from build123d import *

# Parameters (mm, degrees)
SKETCH_W             = 133
SKETCH_H             = 90
PAD_DEPTH            = 10
PAD001_DEPTH         = 24
PAD002_DEPTH         = 133
SKETCH003_W          = 101
SKETCH003_H          = 2
PAD003_DEPTH         = 36
SKETCH004_W          = 2
SKETCH004_H          = 3
PAD004_DEPTH         = 30
LINEARPATTERN_COUNT  = 6
LINEARPATTERN_PITCH  = 16.6
SKETCH005_W          = 100
SKETCH005_H          = 55
POCKET_DEPTH         = 6
SKETCH006_W          = 94
SKETCH006_H          = 49
POCKET001_DEPTH      = 36.001
SKETCH007_W          = 6
SKETCH007_H          = 6
POCKET002_DEPTH      = 57
POCKET002_DEPTH_BACK = -57
FILLET_R             = 3
FILLET001_R          = 3
CHAMFER_SIZE         = 1
SKETCH008_W          = 3
SKETCH008_H          = 55
PAD005_DEPTH         = 3
FILLET002_R          = 2
FILLET003_R          = 2


with BuildPart() as part:
    # Sketch → Pad (new body)
    with BuildSketch(Plane.XY):
        with Locations((0, 5)):
            Rectangle(SKETCH_W, SKETCH_H)
    extrude(amount=PAD_DEPTH)

    # Sketch001 → Pad001 (join)
    with BuildSketch(Plane.XY):
        with BuildLine():
            Line((-66.5, -40), (-66.5, 50))
            Line((-66.5, 50), (-54, 50))
            Line((-54, 50), (-54, 48))
            Line((-54, 48), (-57, 48))
            Line((-57, 48), (-57, 42))
            Line((-57, 42), (-54, 42))
            Line((-54, 42), (-54, 40))
            Line((-54, 40), (-57, 40))
            Line((-57, 40), (-57, -32))
            Line((-57, -32), (-55.06066, -33.93934))
            ThreePointArc((-55.06066, -36.06066), (-54.62132, -35), (-55.06066, -33.93934))
            Line((-55.06066, -36.06066), (-57, -38))
            Line((-57, -38), (-57, -40))
            Line((-57, -40), (-66.5, -40))
        make_face()
    pad001 = extrude(amount=PAD001_DEPTH)

    # Mirrored: Pad001 across Sketch001 V_Axis
    add(pad001.mirror(Plane(origin=(0, 0, 0), x_dir=(0, 0, 1), z_dir=(1, 0, 0))))

    # Sketch002 (on Face10 of Mirrored) → Pad002 (join)
    with BuildSketch(Plane(origin=(-66.5, 0, 0), x_dir=(0, -1, 0), z_dir=(-1, 0, 0))):
        with BuildLine():
            Line((32, 10), (33.93934, 11.93934))
            ThreePointArc((36.06066, 11.93934), (35, 12.37868), (33.93934, 11.93934))
            Line((36.06066, 11.93934), (38, 10))
            Line((38, 10), (32, 10))
        make_face()
    extrude(amount=-PAD002_DEPTH)

    # Sketch003 → Pad003 (join)
    with BuildSketch(Plane.XY):
        with Locations((0, -26.5)):
            Rectangle(SKETCH003_W, SKETCH003_H)
    extrude(amount=PAD003_DEPTH)

    # Sketch004 → Pad004 (join)
    with BuildSketch(Plane.XY):
        with Locations((41.6, -24.5)):
            Rectangle(SKETCH004_W, SKETCH004_H)
    pad004 = extrude(amount=PAD004_DEPTH)

    # LinearPattern: Pad004 ×6
    with Locations(*[(-i * LINEARPATTERN_PITCH, 0, 0) for i in range(1, LINEARPATTERN_COUNT)]):
        add(pad004)

    # Sketch005 (on Face38 of LinearPattern) → Pocket (cut)
    with BuildSketch(Plane.XY.offset(10)):
        with Locations((0, 7.5)):
            Rectangle(SKETCH005_W, SKETCH005_H)
    extrude(amount=-POCKET_DEPTH, mode=Mode.SUBTRACT)

    # Sketch006 → Pocket001 (cut, through all)
    with BuildSketch(Plane.XY):
        with Locations((0, 7.5)):
            Rectangle(SKETCH006_W, SKETCH006_H)
    extrude(amount=POCKET001_DEPTH, mode=Mode.SUBTRACT)

    # Sketch007 → Pocket002 (cut, two sides)
    with BuildSketch(Plane.YZ) as pocket002_sk:
        with Locations((45, 8)):
            Rectangle(SKETCH007_W, SKETCH007_H)
    extrude(amount=-POCKET002_DEPTH, mode=Mode.SUBTRACT)
    extrude(pocket002_sk.sketch, amount=-POCKET002_DEPTH_BACK, mode=Mode.SUBTRACT)

    # Fillet
    fillet_edges = [part.edges().sort_by_distance(p)[0] for p in [
        (-66.5, -40, 17),
        (-66.5, -40, 5),
        (-66.5, 50, 17),
        (-66.5, 50, 5),
    ]]
    fillet(fillet_edges, radius=FILLET_R)

    # Fillet001
    fillet001_edges = [part.edges().sort_by_distance(p)[0] for p in [
        (66.5, 50, 17),
        (66.5, 50, 5),
        (66.5, -40, 17),
        (66.5, -40, 5),
    ]]
    fillet(fillet001_edges, radius=FILLET001_R)

    # Chamfer
    chamfer_edges = [part.edges().sort_by_distance(p)[0] for p in [
        (66.5, 5, 0),
        (65.62132, 49.12132, 0),
        (58.75, 50, 0),
        (0, 50, 0),
        (-58.75, 50, 0),
        (-65.62132, 49.12132, 0),
        (-66.5, 5, 0),
        (-65.62132, -39.12132, 0),
        (-60.25, -40, 0),
        (0, -40, 0),
        (60.25, -40, 0),
        (65.62132, -39.12132, 0),
    ]]
    chamfer(chamfer_edges, length=CHAMFER_SIZE)

    # Sketch008 (on Face13 of Chamfer) → Pad005 (join)
    with BuildSketch(Plane.XY.offset(24)):
        with Locations((58.5, 7.5)):
            Rectangle(SKETCH008_W, SKETCH008_H)
        with Locations((-58.5, 7.5)):
            Rectangle(SKETCH008_W, SKETCH008_H)
    extrude(amount=PAD005_DEPTH)

    # Fillet002
    fillet002_edges = [part.edges().sort_by_distance(p)[0] for p in [
        (60, -20, 25.5),
        (60, 35, 25.5),
    ]]
    fillet(fillet002_edges, radius=FILLET002_R)

    # Fillet003
    fillet003_edges = [part.edges().sort_by_distance(p)[0] for p in [
        (-60, -20, 25.5),
        (-60, 35, 25.5),
    ]]
    fillet(fillet003_edges, radius=FILLET003_R)


solid = part.part
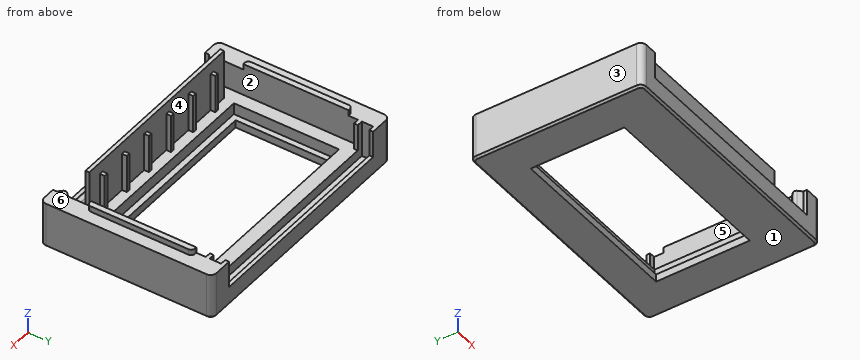
Could you check a few things on this model? Use its own coordinates, in mm. Face numbers are marked on the shaded views. A direction names the side the tool comes from. Coordinates: 2 decimals unless noted, no trailing zeros. Order: outer loops, then holes, each group sorted by start corner. A loop starts at its lowest first (then second) coordinate and runs counter-clockwise, first axis right, second up. Notation, with made-up numbers: (86.25, -22.5) -> (103.25, -22.5) arc R23 cw to (103.25, -14.5) -> close; hole circle Ø3 at (13, 8.25). An arc over 180 degrees is marked (long way). One line per item, written item: value. Start each with the question number.
1) Imagine slicing it at B-B on y = 19. List the corners of the cut face in (x, z) for me.
2) Which directions (+Z, -Z, +X, -X, +Y, -Y) give clear straight access to the entire face, cutting with the end or side of a thin tool? Please do the marked faces 1 and 2.
3) We'd pull the mould along X, two halves only. Please class the marked faces 3, 4, 5 and 6: +X half, -X half, draft (parallel to the pull), parting line (faces both ways), or undercut.
4) I'm going to push flat-ended pins straight in: pin 1 (0.8 mm diameter, centred on x = 57.5, z = 26, fed in from +Y); pin 2 (0.9 mm diameter, centred on x = -58.5, y = 8.5, fed in from +Z); pin 3 (1 mm diameter, centred on x = -41, z = 18.5, fed in from +Y). Where does each tip first touch, or does it pass through?
5) Imagine slicing it at D-D on y = -21.5. List the corners of the cut face in (x, z) for me.
6) Imagine slicing it at C-C on z = 8.5. List the corners of the cut face in (x, y) for me.
7) If I drill on L1, parallel to X at y = -27, z = 22; L2, parallel to X at y = 38.5, z = 22; L3, parallel to X at y = -25, z = 26.5, over which ranges is the centre line in solid material (lowest first)? Write a range as [from, to].
8) Imagine slicing it at A-A on x = 34. List the corners of the cut face in (y, z) for me, plus the area to 3 significant figures.
Answer list:
1. outline: (-66.5, 1) -> (-65.5, 0) -> (-47, 0) -> (-47, 4) -> (-50, 4) -> (-50, 10) -> (-57, 10) -> (-57, 27) -> (-60, 27) -> (-60, 24) -> (-66.5, 24) -> close; (47, 0) -> (65.5, 0) -> (66.5, 1) -> (66.5, 24) -> (60, 24) -> (60, 27) -> (57, 27) -> (57, 10) -> (50, 10) -> (50, 4) -> (47, 4) -> close
2. face 1: -Z, +X, -X, +Y, -Y
2. face 2: +Z
3. face 3: -X half
3. face 4: undercut
3. face 5: undercut
3. face 6: draft
4. pin 1: stops at y = 35
4. pin 2: stops at z = 27
4. pin 3: stops at y = -23
5. outline: (-66.5, 1) -> (-65.5, 0) -> (65.5, 0) -> (66.5, 1) -> (66.5, 24) -> (57, 24) -> (57, 10) -> (-57, 10) -> (-57, 24) -> (-66.5, 24) -> close
6. outline: (-66.5, -37) arc R3 ccw to (-63.5, -40) -> (63.5, -40) arc R3 ccw to (66.5, -37) -> (66.5, 47) arc R3 ccw to (63.5, 50) -> (-63.5, 50) arc R3 ccw to (-66.5, 47) -> close; hole (-57, 42) -> (57, 42) -> (57, 48) -> (-57, 48) -> close; hole (-50, -20) -> (50, -20) -> (50, 35) -> (-50, 35) -> close
7. L1: x = [-66.5, -57], [-50.5, 50.5], [57, 66.5]
7. L2: x = [-66.5, -57], [57, 66.5]
7. L3: x = [-42.4, -40.4], [-25.8, -23.8], [-9.2, -7.2], [7.4, 9.4], [24, 26], [40.6, 42.6]
8. outline: (-40, 1) -> (-39, 0) -> (-17, 0) -> (-17, 4) -> (-20, 4) -> (-20, 10) -> (-25.5, 10) -> (-25.5, 36) -> (-27.5, 36) -> (-27.5, 10) -> (-32, 10) -> (-33.94, 11.94) arc R1.5 ccw to (-36.06, 11.94) -> (-38, 10) -> (-40, 10) -> close; (32, 0) -> (49, 0) -> (50, 1) -> (50, 10) -> (48, 10) -> (48, 5) -> (42, 5) -> (42, 10) -> (35, 10) -> (35, 4) -> (32, 4) -> close
8. area: 404 mm2
